Input: dimensioned drawing with shaded views. Units: mm. Origin: part minimum x, y, z. A direction names the side the tool comes from. Give positions to 0.01 mm unless a question says otherwise; leave off trailing zeros. Loops run counter-clockwise (first coordinate to the right, second up) from the corner with the lowest first, then second, coordinate; pieces in that order, holes last. Notation, with made-up numbers: M -39.5,-24.5 L -23.5,-24.5 A30 ccw -23.5,0.5 Z; hole C 29.5,-21.5 d5. An arc over 180 degrees is marked long. One line per question, with ' | ' between items. Start each with the question number.
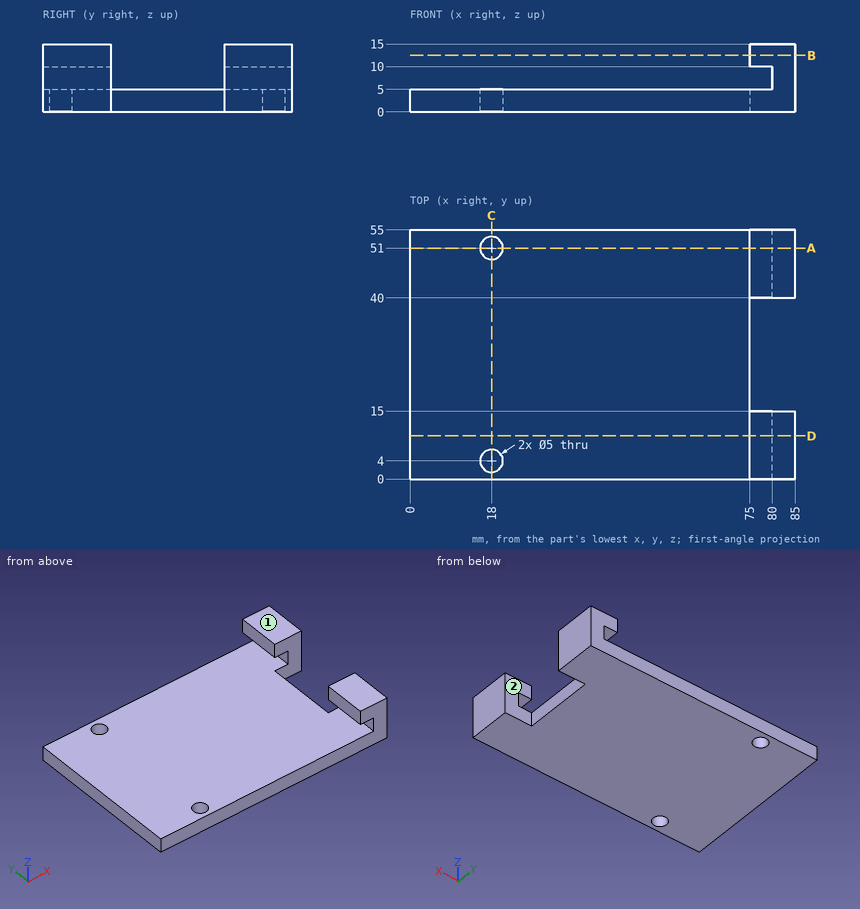
Q1. Section A-A, the plane y = 51. Output: boundary loops of the cut face in (x, z), plus the area to 3 significant figures.
Q2. Section B-B, the plane z = 12.5. Output: boundary loops of the cut face in (x, y).
Q3. Material intervals for L1, parallel to Y at x = 18, z = 2.6; L2, parallel to Y at x = 16, z = 2.25; L3, parallel to Z at x = 10.5, y = 18.5, sorted ascending.
Q4. Section C-C, the plane x = 18. Output: boundary loops of the cut face in (y, z).
Q5. Set-up query: the marked faces 1 and 2. Return all of +Z, -Z, +X, -X, +Y, -Y with unobstructed straight access to the full face (end or side cutting, diameter ignored); none if empty.
Q6. Section D-D, the plane y = 9.5. Output: boundary loops of the cut face in (x, z).
Q7. Contact query for flat-ended pins moving along their axis: pin 1 (2 mm diameter, centred on x = 68.5, y = 39.5, fed in from +Z); pin 2 (4 mm diameter, centred on y = 44.5, z = 12, fed in from -X); pin 3 (2.5 mm diameter, centred on y = 31, z = 3, fed in from +X). Output: stop coordinate, or through.
Model answer:
1) outline: M 0,0 L 15.5,0 L 15.5,5 L 0,5 Z; M 20.5,0 L 85,0 L 85,15 L 75,15 L 75,10 L 80,10 L 80,5 L 20.5,5 Z | area: 475 mm^2
2) outline: M 75,0 L 85,0 L 85,15 L 75,15 Z; M 75,40 L 85,40 L 85,55 L 75,55 Z
3) L1: y = 0 to 1.5, 6.5 to 48.5, 53.5 to 55 | L2: y = 0 to 2.5, 5.5 to 49.5, 52.5 to 55 | L3: z = 0 to 5
4) outline: M 0,0 L 1.5,0 L 1.5,5 L 0,5 Z; M 6.5,0 L 48.5,0 L 48.5,5 L 6.5,5 Z; M 53.5,0 L 55,0 L 55,5 L 53.5,5 Z
5) face 1: +Z, +X, -X, +Y, -Y | face 2: +Z, -Z, +X
6) outline: M 0,0 L 85,0 L 85,15 L 75,15 L 75,10 L 80,10 L 80,5 L 0,5 Z
7) pin 1: stops at z = 5 | pin 2: stops at x = 75 | pin 3: stops at x = 75
